from build123d import *

# Parameters (mm, degrees)
SKETCH1_W           = 14
SKETCH1_H           = 32
SKETCH1_R           = 1.5
BOSS_EXTRUDE1_DEPTH = 7
SKETCH3_R           = 12.5
BOSS_EXTRUDE2_DEPTH = 200
SKETCH4_OUTSIDE_W   = 73.936
SKETCH4_OUTSIDE_H   = 73.936
SKETCH4_OUTSIDE_W_2 = 15
SKETCH4_OUTSIDE_H_2 = 15
CUT_EXTRUDE1_DEPTH  = 10
SKETCH5_R           = 1.5
CUT_EXTRUDE2_DEPTH  = 234.195733237
SKETCH6_R           = 5
CUT_EXTRUDE3_DEPTH  = 233.672516641


with BuildPart() as part:
    # Sketch1 → Boss-Extrude1 (new, symmetric)
    with BuildSketch(Plane.XY):
        with Locations((0, 16)):
            Rectangle(SKETCH1_W, SKETCH1_H)
        with Locations((0, 5)):
            Circle(SKETCH1_R, mode=Mode.SUBTRACT)
        with Locations((0, 25)):
            Circle(SKETCH1_R, mode=Mode.SUBTRACT)
    extrude(amount=BOSS_EXTRUDE1_DEPTH, both=True)

    # Sketch3 → Boss-Extrude2 (add)
    with BuildSketch(Plane(origin=(0, 32, 0), x_dir=(1, 0, 0), z_dir=(0, 1, 0))):
        with Locations(Location((0, 0, 0), (0, 0, 270))):
            Circle(SKETCH3_R)
    extrude(amount=BOSS_EXTRUDE2_DEPTH)

    # Sketch4 outside → Cut-Extrude1 (cut)
    with BuildSketch(Plane(origin=(0, 232, 0), x_dir=(1, 0, 0), z_dir=(0, 1, 0))):
        Rectangle(SKETCH4_OUTSIDE_W, SKETCH4_OUTSIDE_H)
        Rectangle(SKETCH4_OUTSIDE_W_2, SKETCH4_OUTSIDE_H_2, mode=Mode.SUBTRACT)
    extrude(amount=-CUT_EXTRUDE1_DEPTH, mode=Mode.SUBTRACT)

    # Sketch5 → Cut-Extrude2 (cut, through all)
    with BuildSketch(Plane.XY.offset(7.5)):
        with Locations((0, 227)):
            Circle(SKETCH5_R)
    extrude(amount=-CUT_EXTRUDE2_DEPTH, mode=Mode.SUBTRACT)

    # Sketch6 → Cut-Extrude3 (cut, through all)
    with BuildSketch(Plane.XZ):
        Circle(SKETCH6_R)
    extrude(amount=-CUT_EXTRUDE3_DEPTH, mode=Mode.SUBTRACT)


solid = part.part
Work out the finished part from the listing and answer in its coordinate system (mm). A direction names the side the tool comes from. Give positions to 0.01 mm unless a question says otherwise; leave off trailing zeros. Order: outer loops, then holes, each group sorted by start corner. A loop starts at its lowest first (then second) coordinate and runs counter-clockwise, first axis right, second up. Notation, with made-up numbers: (6.5, 22) -> (25.5, 22) arc R22 ccw to (25.5, 45) -> close; hole circle Ø10 at (5.25, -19.5). An arc over 180 degrees is marked (long way). Answer as a JSON object with one key per item and string values. Group by question number.
1. A tool of negligible diameter and unlimited length cuts with its end or side. For faces 5 (the flat face through (-2, 227, 7.5)), 6 (the flat face through (-7, 16, 0)), 7 (the flat face through (0, 16, -7)), from which of +Z, -Z, +X, -X, +Y, -Y can it reach the whole face along a straight path? Write none if from no direction.
2. Section A-A on z = 0 is taken. Determine the outline of the cut face in (x, y), plus the area to 3 significant figures.
3. Section B-B on y = 169 is taken. Determine the outline of the cut face in (x, z).
4. Consider line 1 along Y through (x, z) = (0, -6); line 2 along X through (y, z) = (227, -5.7); line 3 along X through (y, z) = (25, -5.65). Determine where each line is inside the solid, lowest interval first. Write a range as [from, to].
5. The mould has two halves that part along Z. Classify faces 1 (the flat face through (-2, 227, -7.5)), 2 (the flat face through (5, 232, -2)), 3 (the cylindrical face through (-1.08, 114.38, -4.88)), 4 (the cylindrical face through (3.755, 125.67, 11.923)): released by +Z, released by -Z, zero draft, split by the parting line, or undercut.
6. Flat-ended cylindrical pins translate along their axes: pin 1 Ø11 at (x, y) = (1.5, 23) entering from -Z; pin 2 Ø1 at (x, y) = (-9.5, 43.5) entering from -Z; pin 3 Ø2.5 at (x, y) = (0, 227) entering from -Z; pin 4 Ø8 at (y, z) = (228, -3.5) entering from -X. Find the tip coordinate at first contact, or state that the pin passes through.
Result sheet:
{
 "1": {"face 5": "+Z, +X, -X, +Y", "face 6": "+Z, -Z, -X, -Y", "face 7": "-Z, +X, -X, -Y"},
 "2": {"outline": "(-12.5, 32) -> (-7, 32) -> (-7, 0) -> (-5, 0) -> (-5, 232) -> (-7.5, 232) -> (-7.5, 222) -> (-12.5, 222) -> close; (5, 0) -> (7, 0) -> (7, 32) -> (12.5, 32) -> (12.5, 222) -> (7.5, 222) -> (7.5, 232) -> (5, 232) -> close", "area": "3,030 mm^2"},
 "3": {"outline": "circle Ø25 at (0, 0); hole circle Ø10 at (0, 0)"},
 "4": {"line 1": "y = [0, 3.5], [6.5, 23.5], [26.5, 225.5], [228.5, 232]", "line 2": "x = [-7.5, -1.5], [1.5, 7.5]", "line 3": "x = [-7, -1.5], [1.5, 7]"},
 "5": {"face 1": "released by -Z", "face 2": "zero draft", "face 3": "undercut", "face 4": "split by the parting line"},
 "6": {"pin 1": "stops at z = -7", "pin 2": "stops at z = -8.67", "pin 3": "passes through", "pin 4": "stops at x = -7.5"}
}
